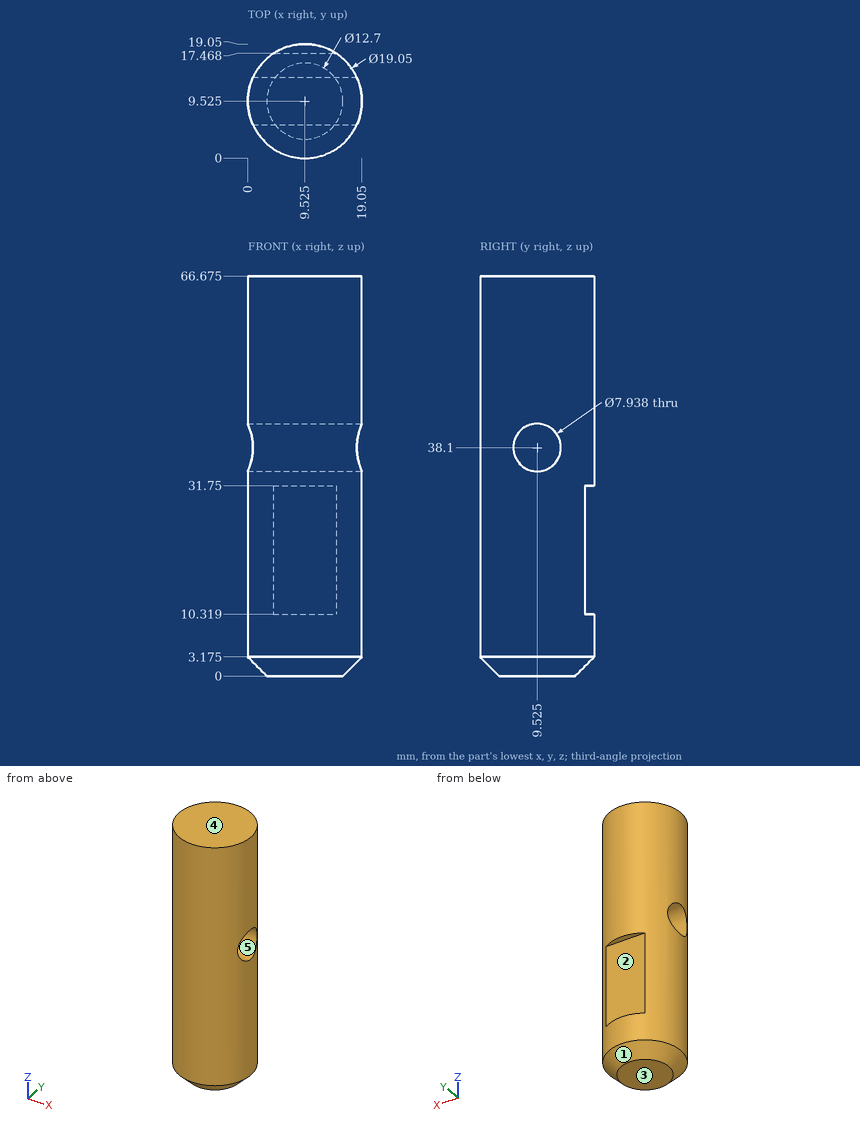
Answer from the drawing. Dimensions are ordinates in mm from the lowest x, y and z of the part. A direction names the side the tool comes from. Round coordinates to 2 decimals unless told otherwise and drop trailing zeros.
1. Which of the six approach directions +Z, -Z, +X, -X, +Y, -Y give full straight-line access (tool end or side, diameter ignored) to the marked faces 1 and 2?
2. Determine the mould class of the marked faces 3, 4 and 5 for opening direction Z: pulls with the +Z half, pulls with the -Z half, needs draft (parallel to the pull), parting line crosses it, or undercut.
3. Straight lines are drawn through the part: L1, parallel to Y at x = 9.5, z = 38.1; L2, parallel to Z at x = 8.5, y = 6 (1 decimal); L3, parallel to Z at x = 3.25, y = 11.25 (1 decimal). For each, find the intervals that lie inside material, in ascending order.
4. Given pin 1 Ø1 at (x, z) = (12, 7) entering from -Y; pin 2 Ø8.5 at (x, z) = (10.5, 20) entering from +Y; pin 3 Ø4 at (y, z) = (2.5, 56) entering from -X, each flat-ended and moving along its own axis, determine where each tip first touches the part or whether it passes through.
Values:
1. face 1: -Z
1. face 2: +X, -X, +Y
2. face 3: pulls with the -Z half
2. face 4: pulls with the +Z half
2. face 5: undercut
3. L1: y = 0 to 5.56, 13.49 to 19.05
3. L2: z = 0 to 36.3, 39.9 to 66.7
3. L3: z = 0.2 to 34.5, 41.7 to 66.7
4. pin 1: stops at y = 0.21
4. pin 2: stops at y = 17.47
4. pin 3: stops at x = 1.43
